Work out the finished part from the listing and answer in its coordinate system (mm). A direction names the side the tool comes from. Coordinates: 2 decimals unless noted, no trailing zeros. Order: outer loops, then holes, each group sorted by start corner. A loop starts at its lowest first (then second) coordinate and runs counter-clockwise, first axis right, second up. Notation, with made-up numbers: M 84.25,58.25 L 120.25,58.25 A16 cw 120.25,77.25 Z; hole C 32,19.5 d5. An arc over 180 degrees is marked long. Answer in a Markdown table with one row per item. Add a question column.
Item 1: Which of the six approach directions +Z, -Z, +X, -X, +Y, -Y give full straight-line access (tool end or side, diameter ignored) to faces 1 (the face through (10, 2, -12)), 2 (the face through (3.753, 3.014, -22.627)), 3 (the face through (5, 2, -8.125))?
Item 2: Consider line 1 (Z direction, x = 5, y = 0.65) (3 decimals); line 2 (Z direction, x = 6.25, y = 1.7) (3 decimals); line 3 (X direction, y = 3.35, z = -21). Determine where each line is inside the solid, lowest interval first. Write a range as from..to.
Item 3: The part is cut by section A-A (x = 5). Write down the section's boundary in (y, z) (3 decimals), then the cut area to 3 significant figures.
Item 4: The part is cut by section D-D (y = 0.75). Write down the section's boundary in (x, z) (3 decimals), then the cut area to 3 significant figures.
Item 5: The part is cut by section C-C (z = -16.5). Write down the section's boundary in (x, y), then the cut area to 3 significant figures.
Item 6: The part is cut by section B-B (y = 3.25). Write down the section's boundary in (x, z) (3 decimals).
Item 7: The mould has two halves that part along X. Classify faces 4 (the face through (5, 0, -12)), 5 (the face through (9.1, 2.03, -0.86)), 6 (the face through (4, 2, -2)): released by +X, released by -X, zero draft, split by the parting line, or undercut.
Item 8: Flat-ended cylindrical pins translate along their axes: pin 1 Ø3 at (x, z) = (5, -21) entering from +Y; pin 2 Ø1.5 at (x, y) = (2, 0.5) entering from +Z. Find the tip coordinate at first contact, or state that the pin passes through.
from build123d import *

# Parameters (mm, degrees)
SKETCH1_W           = 10
SKETCH1_H           = 24
SKETCH1_R           = 1.2
SKETCH1_W_2         = 2.8
SKETCH1_H_2         = 2.4
BOSS_EXTRUDE1_DEPTH = 4
FILLET1_R           = 3
SKETCH2_R           = 2.05
CUT_EXTRUDE1_DEPTH  = 2


with BuildPart() as part:
    # Sketch1 → Boss-Extrude1 (new body)
    with BuildSketch(Plane(origin=(0, 0, 0), x_dir=(1, 0, 0), z_dir=(0, 1, 0))):
        with Locations((5, 12)):
            Rectangle(SKETCH1_W, SKETCH1_H)
        with Locations(Location((5, 21, 0), (0, 0, 270))):
            Circle(SKETCH1_R, mode=Mode.SUBTRACT)
        with Locations(Location((5, 3, 0), (0, 0, 270))):
            Circle(SKETCH1_R, mode=Mode.SUBTRACT)
        with Locations((5, 17.075)):
            Rectangle(SKETCH1_W_2, SKETCH1_H_2, mode=Mode.SUBTRACT)
        with Locations((5, 6.925)):
            Rectangle(SKETCH1_W_2, SKETCH1_H_2, mode=Mode.SUBTRACT)
    extrude(amount=BOSS_EXTRUDE1_DEPTH)

    # Fillet1
    fillet1_edges = [part.edges().sort_by_distance(p)[0] for p in [
        (0, 2, -24),
        (10, 2, -24),
        (10, 2, 0),
        (0, 2, 0),
    ]]
    fillet(fillet1_edges, radius=FILLET1_R)

    # Sketch2 → Cut-Extrude1 (cut)
    with BuildSketch(Plane(origin=(0, 4, 0), x_dir=(1, 0, 0), z_dir=(0, 1, 0))):
        with Locations(Location((5, 3, 0), (0, 0, 270))):
            Circle(SKETCH2_R)
        with Locations(Location((5, 21, 0), (0, 0, 270))):
            Circle(SKETCH2_R)
    extrude(amount=-CUT_EXTRUDE1_DEPTH, mode=Mode.SUBTRACT)


solid = part.part
Reply:
| question | item | result |
|---|---|---|
| 1 | face 1 | +Z, -Z, +X, +Y, -Y |
| 1 | face 2 | +Y |
| 1 | face 3 | +Y, -Y |
| 2 | line 1 | z = -24..-22.2, -19.8..-18.275, -15.875..-8.125, -5.725..-4.2, -1.8..0 |
| 2 | line 2 | z = -24..-18.275, -15.875..-8.125, -5.725..0 |
| 2 | line 3 | x = 0..2.95, 7.05..10 |
| 3 | outline | M 0,-24 L 4,-24 L 4,-23.05 L 2,-23.05 L 2,-22.2 L 0,-22.2 Z; M 0,-19.8 L 2,-19.8 L 2,-18.95 L 4,-18.95 L 4,-18.275 L 0,-18.275 Z; M 0,-15.875 L 4,-15.875 L 4,-8.125 L 0,-8.125 Z; M 0,-5.725 L 4,-5.725 L 4,-5.05 L 2,-5.05 L 2,-4.2 L 0,-4.2 Z; M 0,-1.8 L 2,-1.8 L 2,-0.95 L 4,-0.95 L 4,0 L 0,0 Z |
| 3 | area | 50.8 mm2 |
| 4 | outline | M 0,-21 A3 ccw 3,-24 L 7,-24 A3 ccw 10,-21 L 10,-3 A3 ccw 7,0 L 3,0 A3 ccw 0,-3 Z; hole M 3.6,-18.275 L 6.4,-18.275 L 6.4,-15.875 L 3.6,-15.875 Z; hole M 3.6,-8.125 L 6.4,-8.125 L 6.4,-5.725 L 3.6,-5.725 Z; hole C 5,-21 d2.4; hole C 5,-3 d2.4 |
| 4 | area | 210 mm2 |
| 5 | outline | M 0,0 L 3.6,0 L 3.6,4 L 0,4 Z; M 6.4,0 L 10,0 L 10,4 L 6.4,4 Z |
| 5 | area | 28.8 mm2 |
| 6 | outline | M 0,-21 A3 ccw 3,-24 L 7,-24 A3 ccw 10,-21 L 10,-3 A3 ccw 7,0 L 3,0 A3 ccw 0,-3 Z; hole C 5,-21 d4.1; hole C 5,-3 d4.1; hole M 3.6,-18.275 L 6.4,-18.275 L 6.4,-15.875 L 3.6,-15.875 Z; hole M 3.6,-8.125 L 6.4,-8.125 L 6.4,-5.725 L 3.6,-5.725 Z |
| 7 | face 4 | zero draft |
| 7 | face 5 | released by +X |
| 7 | face 6 | undercut |
| 8 | pin 1 | stops at y = 2 |
| 8 | pin 2 | stops at z = -0.01 |
